Part model, mm, in its own coordinate system. A direction names the side the tool comes from. Give positions to 0.01 mm unless a question says otherwise; leave off trailing zeros. Write each loop counter-clockwise with the first axis right and the second up, starting at its lowest first coordinate (ties: lowest second). Pieces come first, ordered by that corner, then holes.
```python
from build123d import *

# Parameters (mm, degrees)
SKETCH1_R           = 8.5
BOSS_EXTRUDE1_DEPTH = 5
FILLET3_R           = 1


with BuildPart() as part:
    # Sketch1 → Boss-Extrude1 (new body)
    with BuildSketch(Plane(origin=(0, 0, 0), x_dir=(1, 0, 0), z_dir=(0, 1, 0))):
        Circle(SKETCH1_R)
        with BuildLine():
            Line((-1.332, 6.504006227), (-1.332, 4.704006227))
            Line((-1.332, 4.704006227), (1.33, 4.704006227))
            Line((1.33, 4.704006227), (1.33, 6.5044155))
            ThreePointArc((1.33, 6.5044155), (0.001020723, -6.638999922), (-1.332, 6.504006227))
        make_face(mode=Mode.SUBTRACT)
    extrude(amount=BOSS_EXTRUDE1_DEPTH)

    # Fillet3
    fillet3_edges = [part.edges().sort_by_distance(p)[0] for p in [
        (-8.5, 0, 0),
    ]]
    fillet(fillet3_edges, radius=FILLET3_R)


solid = part.part
```
1) Two-plate mould, pull along Z, no slides. Class faces 1 (the face through (0, 0, -5)), 2 (the face through (4.57, 2.972, -7.167)), 3 (the face through (0, 2, -4.704)): +Z half, -Z half, draft (parallel to the pull), parting line (faces both ways), or undercut.
Answers follow:
face 1: draft
face 2: parting line
face 3: undercut
2) Saw through at B-B, the plane z = 0. Write the cut outline in (x, y), then the cut area to 3 significant figures.
Answers follow:
outline: (-8.5, 1) arc R1 ccw to (-7.5, 0) - (-6.64, 0) - (-6.64, 5) - (-8.5, 5) - close; (6.64, 0) - (7.5, 0) arc R1 ccw to (8.5, 1) - (8.5, 5) - (6.64, 5) - close
area: 18.2 mm2
3) Saw through at A-A, the plane x = 0. Write the cut outline in (y, z), then the cut area to 3 significant figures.
Answers follow:
outline: (0, -7.5) arc R1 ccw to (1, -8.5) - (5, -8.5) - (5, -4.7) - (0, -4.7) - close; (0, 6.64) - (5, 6.64) - (5, 8.5) - (1, 8.5) arc R1 ccw to (0, 7.5) - close
area: 27.9 mm2
4) 3-axis set-ups, long thin cutter, end or side, ignore diameter. For faces 4 (the face through (-1.332, 2, -6)), 5 (the face through (0, 5, -5)): which of +Z, -Z, +X, -X, +Y, -Y reach the whole face in a straight line?
Answers follow:
face 4: +Y, -Y
face 5: +Z, -Z, +X, -X, +Y
5) Wall check: L1, parallel to Z at x = 0, y = 2.3; L2, parallel to X at y = 2.9, z = 0; L3, parallel to X at y = 3.7, z = 2.75. Give the ranges that are in metal, low to high.
Answers follow:
L1: z = -8.5 to -4.7, 6.64 to 8.5
L2: x = -8.5 to -6.64, 6.64 to 8.5
L3: x = -8.04 to -6.04, 6.04 to 8.04
6) Saw through at C-C, the plane y = 3.4. Write the cut outline in (x, z).
Answers follow:
outline: circle Ø17 at (0, 0); hole (-1.33, -6.5) - (-1.33, -4.7) - (1.33, -4.7) - (1.33, -6.5) arc R6.64 ccw (long way) to start
7) Pin check, flat tips, straight feed: pin 1 Ø10 at (x, z) = (0, -2) entering from +Y; pin 2 Ø3 at (y, z) = (2.5, 6) entering from +X; pin 3 Ø2 at (x, y) = (4.5, 4) entering from +Z; pin 4 Ø2 at (y, z) = (3, -6) entering from +X. Stop position of each tip, or through.
Answers follow:
pin 1: stops at y = 5
pin 2: stops at x = 7.21
pin 3: stops at z = 7.75
pin 4: stops at x = 6.87
